```python
from build123d import *

# Parameters (mm, degrees)
SKETCH1_W           = 101.6
SKETCH1_H           = 101.6
BOSS_EXTRUDE1_DEPTH = 6.35
SKETCH2_W           = 44.45
SKETCH2_H           = 9.525
BOSS_EXTRUDE2_DEPTH = 50.8
SKETCH3_R           = 6.35
CUT_EXTRUDE1_DEPTH  = 74.025


with BuildPart() as part:
    # Sketch1 → Boss-Extrude1 (new body)
    with BuildSketch(Plane(origin=(0, 0, 0), x_dir=(0, -1, 0), z_dir=(1, 0, 0))):
        Rectangle(SKETCH1_W, SKETCH1_H)
    extrude(amount=BOSS_EXTRUDE1_DEPTH)

    # Sketch2 → Boss-Extrude2 (add)
    with BuildSketch(Plane(origin=(6.35, 0, 0), x_dir=(0, -1, 0), z_dir=(1, 0, 0))):
        with Locations((0, 17.4625)):
            Rectangle(SKETCH2_W, SKETCH2_H)
        with Locations((0, -17.4625)):
            Rectangle(SKETCH2_W, SKETCH2_H)
    extrude(amount=BOSS_EXTRUDE2_DEPTH)

    # Sketch3 → Cut-Extrude1 (cut, through all)
    with BuildSketch(Plane.YX.offset(22.225)):
        with BuildLine():
            Line((-22.225, 57.15), (-22.225, 34.925))
            ThreePointArc((-22.225, 34.925), (-15.715448108, 50.640448315), (2.93e-07, 57.15))
            Line((2.93e-07, 57.15), (-22.225, 57.15))
        make_face()
        with BuildLine():
            ThreePointArc((2.93e-07, 57.15), (15.715448315, 50.640448108), (22.225, 34.925))
            Line((22.225, 34.925), (22.225, 57.15))
            Line((22.225, 57.15), (2.93e-07, 57.15))
        make_face()
        with Locations((0, 34.925)):
            Circle(SKETCH3_R)
    extrude(amount=-CUT_EXTRUDE1_DEPTH, mode=Mode.SUBTRACT)


solid = part.part
```
Input: part model. Units: mm. Frame: model coordinates. A direction names the side the tool comes from. Coordinates: 2 decimals unless noted, no trailing zeros. Write each loop counter-clockwise with the first axis right and the second up, starting at its lowest first coordinate (ties: lowest second). Pieces come first, ordered by that corner, then holes.
1) Section B-B on y = 4.5. Output: boundary loops of the cut face in (x, z) (3 decimals), and give its area (3 significant figures).
2) Section A-A on z = 19. Output: boundary loops of the cut face in (x, y) (3 decimals).
3) Set-up query: faces 1 (the flat face through (26, 0, 22.225)), 2 (the flat face through (20, 22.225, -17)), 3 (the flat face through (20, -22.225, -17)). Return all of +Z, -Z, +X, -X, +Y, -Y with unobstructed straight access to the full face (end or side cutting, diameter ignored); none if empty.
4) Mould query, pull axis X, two halves, no side actions, for faces 4 (the cylindrical face through (41.22, -0.83, 17.4)), 5 (the flat face through (26, 0, -22.225)), 6 (the flat face through (0, 1, -1)), 7 (the cylindrical face through (41.22, -0.83, -17.53)). Classes: pulls with the +X half, pulls with the -X half, needs draft (parallel to the pull), parting line crosses it, or undercut.
5) Pin query (flat end, axial travel): pin 1 Ø7.5 at (x, z) = (25.5, 19) entering from -Y (3 decimals); pin 2 Ø3 at (x, z) = (23, 16) entering from +Y (3 decimals); pin 3 Ø1 at (y, z) = (36.5, -36.5) entering from +X; pin 4 Ø7.5 at (x, y) = (34.925, 0) entering from -Z. Return the tip coordinate at first contact, or that it passes through.
6) Section D-D on y = -19.5. Output: boundary loops of the cut face in (x, z) (3 decimals).
7) Section C-C on z = 1. Output: boundary loops of the cut face in (x, y).
8) Material intervals for line 1 along X through (y, z) = (12, 43); line 2 along Z through (x, y) = (44, 9) (3 decimals); line 3 along Y through (x, z) = (21.5, -19) (3 decimals), sorted ascending.
Check result:
1. outline: (0, -50.8) - (6.35, -50.8) - (6.35, -22.225) - (30.445, -22.225) - (30.445, -12.7) - (6.35, -12.7) - (6.35, 12.7) - (30.445, 12.7) - (30.445, 22.225) - (6.35, 22.225) - (6.35, 50.8) - (0, 50.8) - close; (39.405, -22.225) - (56.69, -22.225) - (56.69, -12.7) - (39.405, -12.7) - close; (39.405, 12.7) - (56.69, 12.7) - (56.69, 22.225) - (39.405, 22.225) - close
1. area: 1,430 mm2
2. outline: (0, -50.8) - (6.35, -50.8) - (6.35, -22.225) - (34.925, -22.225) arc R22.225 ccw to (34.925, 22.225) - (6.35, 22.225) - (6.35, 50.8) - (0, 50.8) - close; hole circle Ø12.7 at (34.925, 0)
3. face 1: +Z, +X, +Y, -Y
3. face 2: +Z, -Z, +X, +Y
3. face 3: +Z, -Z, +X, -Y
4. face 4: undercut
4. face 5: needs draft
4. face 6: pulls with the -X half
4. face 7: undercut
5. pin 1: stops at y = -22.225
5. pin 2: stops at y = 22.225
5. pin 3: stops at x = 6.35
5. pin 4: passes through
6. outline: (0, -50.8) - (6.35, -50.8) - (6.35, -22.225) - (45.588, -22.225) - (45.588, -12.7) - (6.35, -12.7) - (6.35, 12.7) - (45.588, 12.7) - (45.588, 22.225) - (6.35, 22.225) - (6.35, 50.8) - (0, 50.8) - close
7. outline: (0, -50.8) - (6.35, -50.8) - (6.35, 50.8) - (0, 50.8) - close
8. line 1: x = 0 to 6.35
8. line 2: z = -22.225 to -12.7, 12.7 to 22.225
8. line 3: y = -22.225 to 22.225
